Could you check a few things on this drawing? It's one solid part, dimensions in mm from its lowest x, y, z. Coordinates: 2 decimals unless noted, no trailing zeros. Order: outer loops, then holes, each group sorted by start corner. A loop starts at its lowest first (then second) coordinate and runs counter-clockwise, first axis right, second up. Notation, with made-up numbers: (0.25, 86) -> (59.25, 86) arc R24 ccw to (59.25, 112) -> close; hole circle Ø3 at (79.25, -12.75). An arc over 180 degrees is marked (long way). Use a Markdown table: item, result. Add a question column.
1. Suppose I cut it at B-B, the plane z = 27.5. List the corners of the cut face in (x, y) for me (1 decimal).
2. Suppose I cut it at A-A, the plane x = 29.5. List the corners of the cut face in (y, z) for me (1 decimal).
3. If I drill on line 1 along X through (y, z) = (3, 17) (1 decimal); line 2 along X through (y, z) = (0.8, 27); line 3 along Z through (x, y) = (36, 2.15) (1 decimal), over which ranges is the centre line in solid material (lowest first)? Write a range as from..to.
4. Suppose I cut it at C-C, the plane x = 18.5. List the corners of the cut face in (y, z) for me (1 decimal), then the cut area to 3 significant figures.
5. Suppose I cut it at D-D, the plane y = 2.6. State how many separate pieces and enclosed holes the cut face has, then the cut area to 3 significant figures.
6. For pin 1 Ø1 at (y, z) = (1, 19) entering from +X; pin 2 Ø6 at (x, z) = (44, 64) entering from -Y; pin 3 Ø1.5 at (x, z) = (15, 13) entering from -Y; pin 4 Ø1 at (x, y) = (32.5, 0.5) entering from +Z, each with a flat end and sliding along its axis, tell me the tip position at first contact or that it passes through.
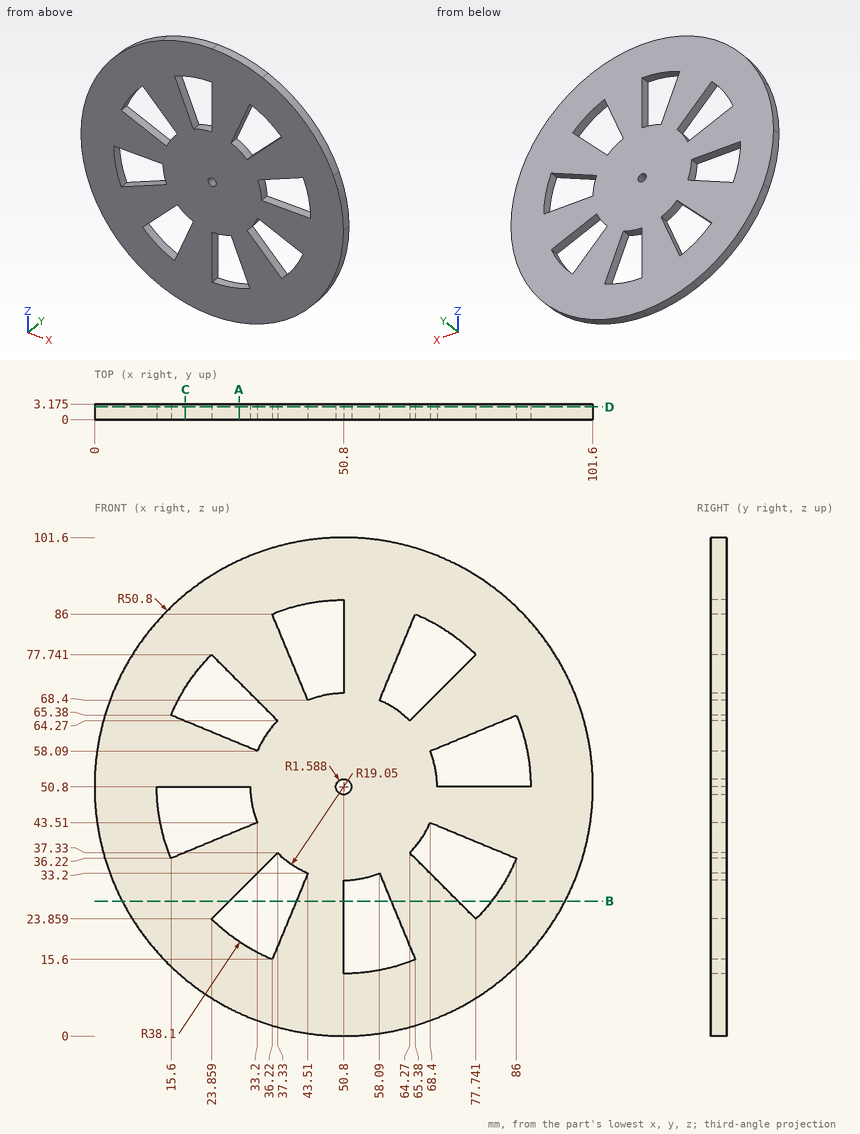
Worked out:
| question | item | result |
|---|---|---|
| 1 | outline | (5.7, 0) -> (27.5, 0) -> (27.5, 3.2) -> (5.7, 3.2) -> close; (41.1, 0) -> (50.8, 0) -> (50.8, 3.2) -> (41.1, 3.2) -> close; (60.5, 0) -> (74.1, 0) -> (74.1, 3.2) -> (60.5, 3.2) -> close; (80.9, 0) -> (95.9, 0) -> (95.9, 3.2) -> (80.9, 3.2) -> close |
| 2 | outline | (0, 4.7) -> (3.2, 4.7) -> (3.2, 19.2) -> (0, 19.2) -> close; (0, 29.5) -> (3.2, 29.5) -> (3.2, 42) -> (0, 42) -> close; (0, 50.8) -> (3.2, 50.8) -> (3.2, 59.6) -> (0, 59.6) -> close; (0, 72.1) -> (3.2, 72.1) -> (3.2, 96.9) -> (0, 96.9) -> close |
| 3 | line 1 | x = 12.9..33.2, 36.8..50.8, 64.8..88.7 |
| 3 | line 2 | x = 5.92..27, 40.94..50.8, 60.66..74.6, 80.55..95.68 |
| 3 | line 3 | z = 2.2..15.7, 36..62.8, 65.6..99.4 |
| 4 | outline | (0, 11.6) -> (3.2, 11.6) -> (3.2, 37.4) -> (0, 37.4) -> close; (0, 50.8) -> (3.2, 50.8) -> (3.2, 64.2) -> (0, 64.2) -> close; (0, 71) -> (3.2, 71) -> (3.2, 90) -> (0, 90) -> close |
| 4 | area | 185 mm² |
| 5 | separate pieces | 1 |
| 5 | enclosed holes | 9 |
| 5 | area | 6,390 mm² |
| 6 | pin 1 | stops at x = 90.81 |
| 6 | pin 2 | stops at y = 0 |
| 6 | pin 3 | passes through |
| 6 | pin 4 | stops at z = 98.38 |
